Model file for the job. Use its own axes, mm. A direction names the side the tool comes from. Coordinates: 2 decimals unless noted, no trailing zeros. Order: outer loops, then holes, each group sorted by start corner. A loop starts at its lowest first (then second) coordinate and runs counter-clockwise, first axis right, second up. Notation, with made-up numbers: (22, -12.75) -> (50, -12.75) arc R33 cw to (50, 15.25) -> close; hole circle Ø6 at (-22, 48.25). An arc over 180 degrees is marked (long way). Write item = value, one per line. Start each with the question number.
Q1. 3-axis set-ups, long thin cutter, end or side, ignore diameter. For faces 5 (the face through (5, 0, -2)), 6 (the face through (2.535, 35.278, -1.972)), 7 (the face through (99.35, 27.95, 1.97)): which of +Z, -Z, +X, -X, +Y, -Y reach the whole face in a straight line?
Q2. Wall check: line 1 (Y direction, x = 129, z = 1.7); line 2 (X direction, y = 12, z = 0.75); line 3 (Z direction, x = 8, y = 4.5). Give the ranges that are in metal, low to high. Write a range as from..to.
Q3. Flat gauge pin, fed straight in: pin 1 (1 mm diameter, centred on x = 68.5, z = -2, fed in from -Y). Where does the tip first touch, or does it go through?
Q4. Cut at A-A, the plane x = 129. List the corners of the cut face in (y, z).
Q5. Cut at C-C, the plane x = 44. List the corners of the cut face in (y, z), plus the area to 3 significant figures.
Q6. Cut at B-B, the plane y = 7.5. List the corners of the cut face in (x, z), plus the area to 3 significant figures.
Q7. Cut at D-D, the plane x = 111.5. List the corners of the cut face in (y, z), plus the area to 4 significant figures.
Q8. Mould opens along Y. For faces 1 (the face through (102, 0, 2)), 2 (the face through (60.8, 47.6, 2)), 3 (the face through (137, -55, 2)), 4 (the face through (0, 1, 0)) say: +Y half, -Y half, draft (parallel to the pull), parting line (faces both ways), or undercut.
from build123d import *

# Parameters (mm, degrees)
F0_R     = 2
F1_DEPTH = 4
F3_DEPTH = 4


with BuildPart() as f1:
    # F0 (on Top) → F1 (new body)
    with BuildSketch(Plane.XY):
        Polygon((120, 55), (0, 40), (0, -40), (120, -55), (155, -55), (155, 55), align=None)
        with BuildLine():
            Line((20, -16.5), (20, 16.5))
            ThreePointArc((20, 16.5), (22.112942, 21.916876), (27.335636, 24.472366))
            Line((27.335636, 24.472366), (93.335636, 29.972366))
            ThreePointArc((93.335636, 29.972366), (99.416876, 27.887058), (102, 22))
            Line((102, 22), (102, -22))
            ThreePointArc((102, -22), (99.416876, -27.887058), (93.335636, -29.972366))
            Line((93.335636, -29.972366), (27.335636, -24.472366))
            ThreePointArc((27.335636, -24.472366), (22.112942, -21.916876), (20, -16.5))
        make_face(mode=Mode.SUBTRACT)
        with Locations((129, 0)):
            Circle(F0_R, mode=Mode.SUBTRACT)
    extrude(amount=F1_DEPTH)

    # F2 (on face) → F3 (join)
    with BuildSketch(Plane.XY):
        Polygon((0, 34.961089), (0, -34.961089), (5, -35.586089), (5, 35.586089), align=None)
    extrude(amount=-F3_DEPTH)


solid = f1.part
Here are the results:
q1.face_5 = -Z, +X, +Y, -Y
q1.face_6 = -Z, -X, +Y
q1.face_7 = +Z, -Z
q2.line_1 = -55..-2, 2..55
q2.line_2 = 0..20, 102..155
q2.line_3 = 0..4
q3.pin_1 = through
q4.outline = (-55, 0) -> (-2, 0) -> (-2, 4) -> (-55, 4) -> close; (2, 0) -> (55, 0) -> (55, 4) -> (2, 4) -> close
q5.outline = (-45.5, 0) -> (-25.86, 0) -> (-25.86, 4) -> (-45.5, 4) -> close; (25.86, 0) -> (45.5, 0) -> (45.5, 4) -> (25.86, 4) -> close
q5.area = 157 mm²
q6.outline = (0, -4) -> (5, -4) -> (5, 0) -> (20, 0) -> (20, 4) -> (0, 4) -> close; (102, 0) -> (155, 0) -> (155, 4) -> (102, 4) -> close
q6.area = 312 mm²
q7.outline = (-53.94, 0) -> (53.94, 0) -> (53.94, 4) -> (-53.94, 4) -> close
q7.area = 431.5 mm²
q8.face_1 = undercut
q8.face_2 = +Y half
q8.face_3 = -Y half
q8.face_4 = draft
